Geometry check sheet. Reference: drawing and pictorial views, mm from the part's lowest x, y, z. A direction names the side the tool comes from. Round coordinates to 2 decimals unless told otherwise and drop trailing zeros. Write each loop counter-clockwise with the first axis right and the second up, starting at its lowest first coordinate (ties: lowest second). Pieces come first, ordered by that corner, then holes. Notation, with made-up numbers: M -30.75,75.5 L 11.25,75.5 A18 cw 11.25,100.5 Z; hole C 31.25,-4.5 d9. An arc over 180 degrees is marked long. Answer in a Markdown table with one row per item. Add a question column.
1. Material ranges on probe 1 along Z at (x, y) = (35, 25.6); probe 2 along Y at (x, z) = (28, 10); probe 3 along X at (y, z) = (0.9, 5), recorded low to high.
2. Set-up check for the marked faces 1, 2 and 3: record each of +Z, -Z, +X, -X, +Y, -Y from which the full face is reachable in a straight line by a thin tool's end or side.
3. Draft check along Y on the marked faces 4, 5 and 6. Enter one of: pulls with the +Y half, pulls with the -Y half, needs draft (parallel to the pull), parting line crosses it, or undercut.
4. Sectioned sample at C-C on y = 2. Record the cut outline in (x, z), plus the area to 3 significant figures.
5. Sectioned sample at A-A on x = 35. Record the cut outline in (y, z).
6. Sectioned sample at B-B on z = 5. Record the cut outline in (x, y), plus the area to 3 significant figures.
7. Go/stop test with flat-tipped pins: pin 1 Ø10 at (x, y) = (32.5, 12) entering from +Z; pin 2 Ø10 at (x, z) = (7.5, 8.5) entering from +Y; pin 3 Ø4.5 at (y, z) = (1.5, 10.5) entering from -X; pin 4 Ø10 at (y, z) = (9.5, 13) entering from +X. Record where each tip stops, or that it passes through.
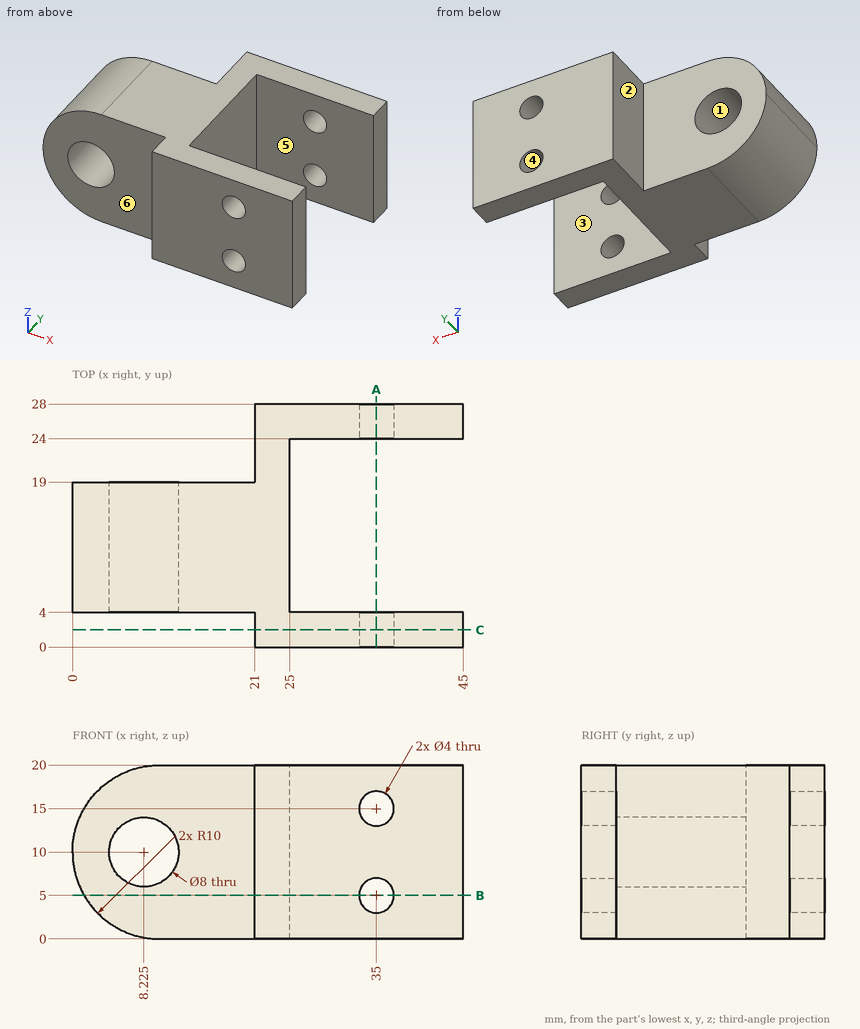
Geometry check:
| question | item | result |
|---|---|---|
| 1 | probe 1 | z = 0 to 3, 7 to 13, 17 to 20 |
| 1 | probe 2 | y = 0 to 4, 24 to 28 |
| 1 | probe 3 | x = 21 to 33, 37 to 45 |
| 2 | face 1 | +Y, -Y |
| 2 | face 2 | +Z, -Z, -X, +Y |
| 2 | face 3 | +Z, -Z, +X |
| 3 | face 4 | needs draft |
| 3 | face 5 | undercut |
| 3 | face 6 | pulls with the -Y half |
| 4 | outline | M 21,0 L 45,0 L 45,20 L 21,20 Z; hole C 35,5 d4; hole C 35,15 d4 |
| 4 | area | 455 mm2 |
| 5 | outline | M 0,0 L 4,0 L 4,3 L 0,3 Z; M 0,7 L 4,7 L 4,13 L 0,13 Z; M 0,17 L 4,17 L 4,20 L 0,20 Z; M 24,0 L 28,0 L 28,3 L 24,3 Z; M 24,7 L 28,7 L 28,13 L 24,13 Z; M 24,17 L 28,17 L 28,20 L 24,20 Z |
| 6 | outline | M 1.34,4 L 21,4 L 21,0 L 33,0 L 33,4 L 25,4 L 25,24 L 33,24 L 33,28 L 21,28 L 21,19 L 1.34,19 Z; M 37,0 L 45,0 L 45,4 L 37,4 Z; M 37,24 L 45,24 L 45,28 L 37,28 Z |
| 6 | area | 535 mm2 |
| 7 | pin 1 | passes through |
| 7 | pin 2 | stops at y = 19 |
| 7 | pin 3 | stops at x = 21 |
| 7 | pin 4 | stops at x = 25 |
